Can you work these out from the drawing? Everything is in mm from the part's minimum corner. A direction names the side the tool comes from. Round coordinates to 2 decimals unless told otherwise and drop trailing zeros. Write each loop counter-clockwise with the first axis right and the second up, starting at its lowest first coordinate (ties: lowest second). Pieces come first, ordered by that corner, then holes. Notation, with made-up numbers: (80.25, 75) - (93.25, 75) arc R25 ccw to (93.25, 101) - close; hole circle Ø10 at (-34.75, -28). An arc over 180 degrees is marked (long way). One line per item, written item: value. Start each with the question number.
Item 1: For P1, Ø5.5, axis at x = 50.5, y = 10, coming from the +Z side; P2, Ø5.5, axis at y = 20, z = 12, coming from the +X side; P3, Ø11, axis at x = 9, y = 51, coming from the +Z side, each with a flat end and sliding along its axis, tell me the tip position at first contact or that it passes through.
Item 2: For the marked faces 1 and 2, which set-ups out of +Z, -Z, +X, -X, +Y, -Y let a thin tool reach every point of the face, with its end or its side?
Item 3: Imagine slicing it at B-B, the plane y = 44.5. Please give me the cut outline in (x, z).
Item 4: Imagine slicing it at C-C, the plane z = 6. Please give me the cut outline in (x, y), then the cut area to 3 significant figures.
Item 5: Imagine slicing it at D-D, the plane x = 7.5. Please give me the cut outline in (y, z).
Item 6: If I drill on line 1 (Y direction, x = 9, z = 0.5); line 2 (X direction, y = 51, z = 2.45); line 3 (X direction, y = 8.5, z = 2.4), over which ranges is the centre line in solid material (lowest first)?
Item 7: Imagine slicing it at A-A, the plane x = 51. Please give me the cut outline in (y, z), then the cut area to 3 significant figures.
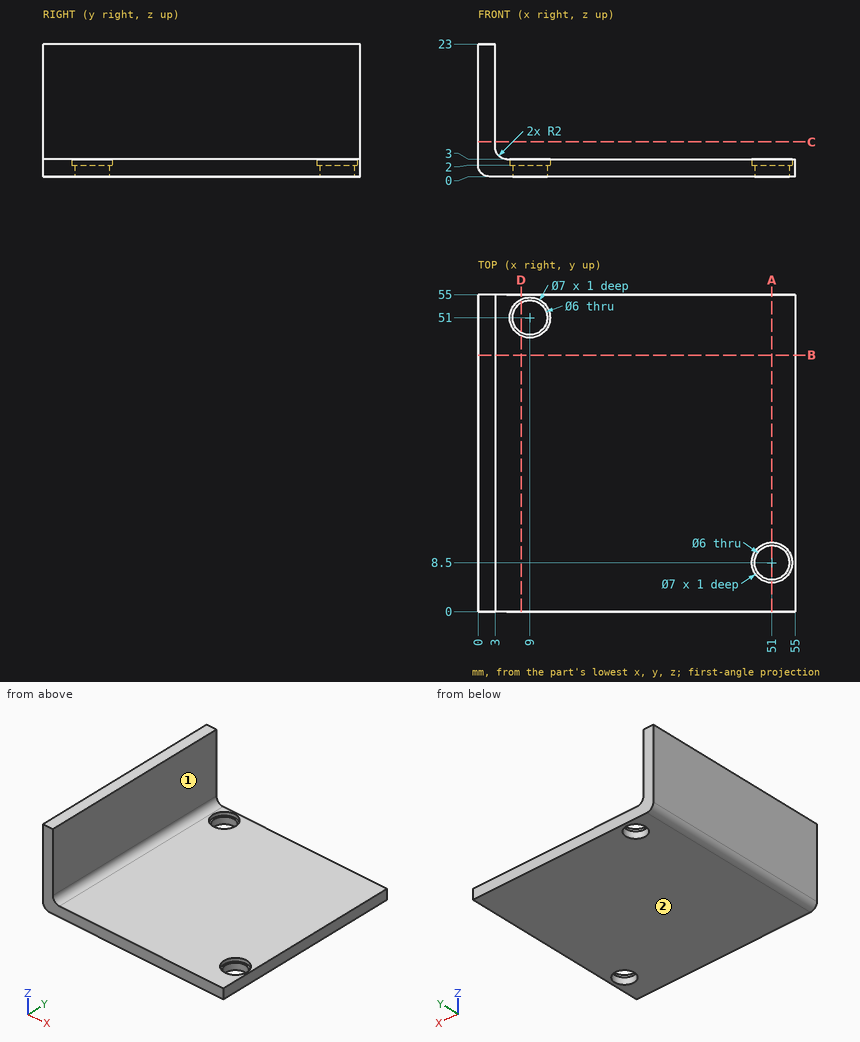
Values follow:
1. P1: stops at z = 3
1. P2: stops at x = 3
1. P3: stops at z = 3.68
2. face 1: +Z, +X, +Y, -Y
2. face 2: -Z, +X, -X, +Y, -Y
3. outline: (0, 2) arc R2 ccw to (2, 0) - (55, 0) - (55, 3) - (5, 3) arc R2 cw to (3, 5) - (3, 23) - (0, 23) - close
4. outline: (0, 0) - (3, 0) - (3, 55) - (0, 55) - close
4. area: 165 mm^2
5. outline: (0, 0) - (48.4, 0) - (48.4, 2) - (47.84, 2) - (47.84, 3) - (0, 3) - close; (53.6, 0) - (55, 0) - (55, 3) - (54.16, 3) - (54.16, 2) - (53.6, 2) - close
6. line 1: y = 0 to 48, 54 to 55
6. line 2: x = 0 to 5.5, 12.5 to 55
6. line 3: x = 0 to 47.5, 54.5 to 55
7. outline: (0, 0) - (5.5, 0) - (5.5, 2) - (5, 2) - (5, 3) - (0, 3) - close; (11.5, 0) - (55, 0) - (55, 3) - (12, 3) - (12, 2) - (11.5, 2) - close
7. area: 146 mm^2
